Autodesk Inventor part; units mm, degrees
ref_plane "YZ Plane" through (0, 0, 0) normal (1, 0, 0) x (0, 1, 0)
ref_plane "XZ Plane" through (0, 0, 0) normal (0, 1, 0) x (-1, 0, 0)
ref_plane "XY Plane" through (0, 0, 0) normal (0, 0, 1) x (1, 0, 0)
sketch "Sketch1" plane through (0, 0, 0) normal (0, 1, 0) x (-1, 0, 0)
  circle A0 centre (0, 0) radius 1.95
  dimension "d0" = 3.9
extrude "Extrusion1" add sketch "Sketch1" along normal blind 16 and the other way blind 7
sketch "Sketch2" plane through (0, 0, 0) normal (0, 1, 0) x (-1, 0, 0)
  circle A0 centre (0, 0) radius 1.95
  circle A1 centre (0, 0) radius 3.45
  dimension "d5" = 1.5
extrude "Extrusion2" add sketch "Sketch2" against normal blind 7
chamfer "Chamfer1" distance 0.5 angle 45 2 edges at (1.95, 16, 0) (3.45, -7, 0)
properties part number "button"
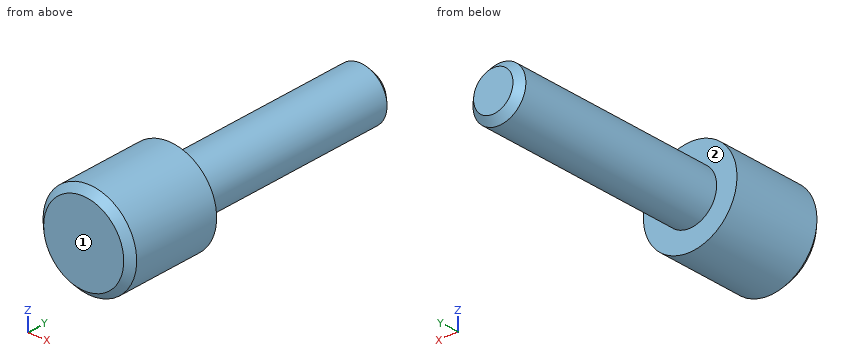
Could you check a few things on this model? Use its own coordinates, in mm. Face numbers are marked on the shaded views. A direction names the side the tool comes from. Give positions to 0.01 mm unless a question says otherwise; leave off trailing zeros. Loops run counter-clockwise (first coordinate to the right, second up) from the corner with the lowest first, then second, coordinate; pieces in that order, holes last. Notation, with made-up numbers: (44, 50.25) -> (56, 50.25) arc R13 ccw to (56, 73.25) -> close; hole circle Ø9 at (23, -10.75). An arc over 180 degrees is marked (long way). Return JSON: item names as keys, results as strings.
Item 1: I'm going to push flat-ended pins straight in: pin 1 (3 mm diameter, centred on y = 5.5, z = 0.5, fed in from +X); pin 2 (4 mm diameter, centred on x = 2.5, y = 7, fed in from +Z); pin 3 (2 mm diameter, centred on x = -1.5, z = 1.5, fed in from +Y). Where does each tip first touch, or does it pass through?
Geometry results:
{"pin 1": "stops at x = 1.95", "pin 2": "stops at z = 1.88", "pin 3": "stops at y = 16"}
Item 2: If we section it at A-A on z = 0: List the corners of the cut face in (x, y) for me, plus the area to 3 significant figures.
Geometry results:
{"outline": "(-3.45, -6.5) -> (-2.95, -7) -> (2.95, -7) -> (3.45, -6.5) -> (3.45, 0) -> (1.95, 0) -> (1.95, 15.5) -> (1.45, 16) -> (-1.45, 16) -> (-1.95, 15.5) -> (-1.95, 0) -> (-3.45, 0) -> close", "area": "110 mm²"}
Item 3: Which directions (+Z, -Z, +X, -X, +Y, -Y) give clear straight access to the entire face, cutting with the end or side of a thin tool? Please do the marked faces 1 and 2.
Geometry results:
{"face 1": "+Z, -Z, +X, -X, -Y", "face 2": "+Y"}
Item 4: I need wall thicknesses on L1, parallel to Y at x = -1.75, z = 2; L2, parallel to Z at x = 0, y = 7; L3, parallel to X at y = -0.75, z = -1.75. Which ranges of each line are inside material? Lowest first, please. Write a range as from..to.
Geometry results:
{"L1": "y = -7..0", "L2": "z = -1.95..1.95", "L3": "x = -2.97..2.97"}
Item 5: If we section it at B-B on x = 0: List the corners of the cut face in (y, z) for me, plus the area to 3 significant figures.
Geometry results:
{"outline": "(-7, -2.95) -> (-6.5, -3.45) -> (0, -3.45) -> (0, -1.95) -> (15.5, -1.95) -> (16, -1.45) -> (16, 1.45) -> (15.5, 1.95) -> (0, 1.95) -> (0, 3.45) -> (-6.5, 3.45) -> (-7, 2.95) -> close", "area": "110 mm²"}
Item 6: If we section it at C-C on y = 8.5: List the corners of the cut face in (x, z) for me.
Geometry results:
{"outline": "circle Ø3.9 at (0, 0)"}
